Check sheet for the modelled part. Datum: model origin and axes. Units: mm. Face numbers are marked on the shaded views. Give positions to 0.01 mm unless a question says otherwise; leave off trailing zeros. Write item = value, one per line. Start each with the question number.
1) Gauge pin test, flat ends, axial feed: pin 1 (5 mm diameter, centred on x = 30, z = 40, fed in from +Y); pin 2 (10 mm diameter, centred on x = -16, z = 19.5, fed in from -Y); pin 3 (6 mm diameter, centred on y = 19, z = 15, fed in from +X). Record the tip position at first contact, or that the pin passes through.
2) Draft check along Y on the marked faces 1, 2 and 3. Enter one of: pulls with the +Y half, pulls with the -Y half, needs draft (parallel to the pull), parting line crosses it, or undercut.
3) Scan lines: L1, parallel to Y at x = -31, z = 16; L2, parallel to X at y = 24.5, z = 39; L3, parallel to X at y = -5, z = 32. Record each from-to range of solid material in increasing order.
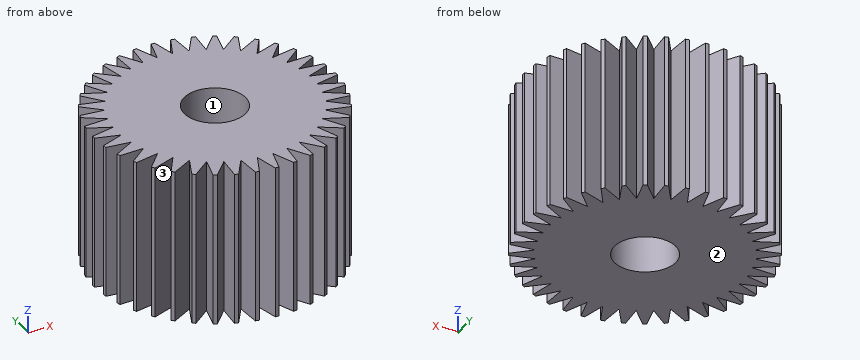
from build123d import *

# Parameters (mm, degrees)
BOSS_EXTRUDE1_DEPTH = 50
SKETCH2_R           = 10
CUT_EXTRUDE1_DEPTH  = 50


with BuildPart() as part:
    # Sketch1 → Boss-Extrude1 (new body)
    with BuildSketch(Plane.XY):
        Polygon((-6.619772583, 31.13494509), (-5.73799784, 38.993038365), (-4.547892767, 39.149686923), (-1.662532106, 31.787453214), (0.437663145, 39.41086036), (1.637621283, 39.379406864), (3.335751275, 31.656444617), (6.602653255, 38.857452051), (7.782917506, 38.638670991), (8.252003232, 30.745145167), (12.605169974, 37.346440186), (13.736678316, 36.945718677), (12.965169329, 29.075994081), (18.297411419, 34.915030894), (19.35230236, 34.342236029), (17.359195772, 26.690091397), (23.539215714, 31.623093539), (24.491514339, 30.892329429), (21.325887048, 23.646185959), (28.201512241, 27.551686544), (29.027769797, 26.680947028), (24.767570054, 20.01922882), (32.169499785, 22.801061463), (32.849371069, 21.811787037), (27.59949913, 15.898527702), (35.345473326, 17.488194451), (35.86221765, 16.404744334), (29.751942786, 11.385547942), (37.651229853, 11.743905927), (37.992123258, 10.592958256), (31.171900714, 6.59141408), (39.029993988, 5.709639337), (39.186642547, 4.519534265), (31.824408837, 1.634173603), (39.447815984, -0.466021647), (39.416362488, -1.665979785), (31.693400241, -3.364109777), (38.894407674, -6.631011757), (38.675626614, -7.811276009), (30.782100791, -8.280361735), (37.38339581, -12.633528476), (36.982674301, -13.765036818), (29.112949705, -12.993527831), (34.951986517, -18.325769921), (34.379191653, -19.380660863), (26.727047021, -17.387554274), (31.660049162, -23.567574216), (30.929285053, -24.519872841), (23.683141582, -21.354245551), (27.588642168, -28.229870743), (26.717902652, -29.056128299), (20.056184443, -24.795928556), (22.838017087, -32.197858288), (21.84874266, -32.877729572), (15.935483325, -27.627857633), (17.525150075, -35.373831828), (16.441699957, -35.890576153), (11.422503566, -29.780301288), (11.78086155, -37.679588355), (10.62991388, -38.02048176), (6.628369704, -31.200259216), (5.746594961, -39.058352491), (4.556489888, -39.215001049), (1.671129227, -31.85276734), (-0.429066024, -39.476174486), (-1.629024161, -39.44472099), (-3.327154153, -31.721758743), (-6.594056134, -38.922766177), (-7.774320385, -38.703985117), (-8.243406111, -30.810459293), (-12.596572853, -37.411754312), (-13.728081194, -37.011032803), (-12.956572207, -29.141308207), (-18.288814298, -34.98034502), (-19.343705239, -34.407550155), (-17.350598651, -26.755405523), (-23.530618592, -31.688407665), (-24.482917218, -30.957643555), (-21.317289927, -23.711500085), (-28.192915119, -27.61700067), (-29.019172675, -26.746261154), (-24.758972932, -20.084542946), (-32.160902664, -22.866375589), (-32.840773948, -21.877101162), (-27.590902009, -15.963841828), (-35.336876204, -17.553508577), (-35.853620529, -16.47005846), (-29.743345665, -11.450862068), (-37.642632731, -11.809220053), (-37.983526136, -10.658272382), (-31.163303592, -6.656728206), (-39.021396867, -5.774953463), (-39.178045425, -4.584848391), (-31.815811716, -1.699487729), (-39.439218862, 0.400707521), (-39.407765367, 1.600665659), (-31.68480312, 3.298795651), (-38.885810553, 6.565697631), (-38.667029493, 7.745961883), (-30.77350367, 8.215047609), (-37.374798689, 12.56821435), (-36.97407718, 13.699722692), (-29.104352583, 12.928213705), (-34.943389396, 18.260455795), (-34.370594532, 19.315346737), (-26.7184499, 17.322240148), (-31.651452041, 23.50226009), (-30.920687932, 24.454558715), (-23.674544461, 21.288931425), (-27.580045047, 28.164556617), (-26.70930553, 28.990814173), (-20.047587322, 24.73061443), (-22.829419966, 32.132544162), (-21.840145539, 32.812415446), (-15.926886204, 27.562543507), (-17.516552954, 35.308517702), (-16.433102836, 35.825262027), (-11.413906444, 29.714987162), (-11.772264429, 37.614274229), (-10.621316758, 37.955167634), align=None)
    extrude(amount=BOSS_EXTRUDE1_DEPTH)

    # Sketch2 → Cut-Extrude1 (cut)
    with BuildSketch(Plane(origin=(0, 0, 0), x_dir=(-1, 0, 0), z_dir=(0, 0, -1))):
        Circle(SKETCH2_R)
    extrude(amount=-CUT_EXTRUDE1_DEPTH, mode=Mode.SUBTRACT)


solid = part.part
Data:
q1.pin_1 = 27.55
q1.pin_2 = -37.41
q1.pin_3 = 35.86
q2.face_1 = undercut
q2.face_2 = needs draft
q2.face_3 = undercut
q3.L1 = -22.43 to -19.8, -16.66 to -12.48, -11.51 to 8.2, 8.36 to 13.11, 14.66 to 18.44, 22.69 to 24.35
q3.L2 = -25.5 to 21.7, 22.83 to 27.63
q3.L3 = -39.12 to -8.66, 8.66 to 35.3
